```python
from build123d import *

# Parameters (mm, degrees)
SKETCH4_W          = 3.175
SKETCH4_H          = 3.175
CUT_EXTRUDE2_DEPTH = 40.272581084
SKETCH5_R          = 1.5875
CUT_EXTRUDE3_DEPTH = 40.272581084
FILLET1_R          = 1.27


with BuildPart() as part:
    # Sketch3 → Revolve2 (revolve)
    with BuildSketch(Plane(origin=(0, 0, 0), x_dir=(0, 0, -1), z_dir=(1, 0, 0)), mode=Mode.PRIVATE) as revolve2_sk:
        Polygon((0, 6.35), (28.575, 6.35), (28.575, 19.05), (26.9875, 19.05), (22.225, 11.1125), (19.05, 11.1125), (14.2875, 19.05), (12.7, 19.05), (12.7, 12.7), (0, 12.7), align=None)
    revolve(revolve2_sk.sketch.rotate(Axis((0, 0, 0), (0, 0, -1)), 90), axis=Axis((0, 0, 0), (0, 0, -1)))

    # Sketch4 → Cut-Extrude2 (cut, through all)
    with BuildSketch(Plane.XY):
        with Locations((0, 6.35)):
            Rectangle(SKETCH4_W, SKETCH4_H)
    extrude(amount=-CUT_EXTRUDE2_DEPTH, mode=Mode.SUBTRACT)

    # Sketch5 → Cut-Extrude3 (cut, through all)
    with BuildSketch(Plane(origin=(0, 0, 0), x_dir=(1, 0, 0), z_dir=(0, 1, 0))):
        with Locations(Location((0, 6.35, 0), (0, 0, 90))):
            Circle(SKETCH5_R)
    extrude(amount=CUT_EXTRUDE3_DEPTH, mode=Mode.SUBTRACT)

    # Fillet1
    fillet1_edges = [part.edges().sort_by_distance(p)[0] for p in [
        (-12.7, 0, -12.7),
        (-12.7, 0, 0),
    ]]
    fillet(fillet1_edges, radius=FILLET1_R)


solid = part.part
```
Geometry: final body of the model. Coordinates: model frame, mm. A direction names the side the tool comes from. Coordinates: 2 decimals unless noted, no trailing zeros. Order: outer loops, then holes, each group sorted by start corner. A loop starts at its lowest first (then second) coordinate and runs counter-clockwise, first axis right, second up. Notation, with made-up numbers: (6, 12) - (53, 12) arc R12 cw to (53, 31) - close; hole circle Ø11 at (73.5, 11.5). An arc over 180 degrees is marked (long way). Return JSON: item names as keys, results as strings. Group by question number.
1. Pull-direction query (Y, two-part tool) for faces 6 (the face through (0, 7.938, -2)), 7 (the face through (1.588, 7, -14)), 8 (the face through (-8.2, -7.5, -20.6)), 9 (the face through (-6, -13, -12.7)); classes: pulls with the +Y half, pulls with the -Y half, needs draft (parallel to the pull), parting line crosses it, or undercut.
2. Set-up query: faces 1 (the face through (-9.124, 6.996, -22.456)), 2 (the face through (-10.1, 7.7, -6.3)), 3 (the face through (0.966, 10.287, -5.09)), 4 (the face through (-1.588, 7, -14)), 5 (the face through (5, -5, -28.575)). Return all of +Z, -Z, +X, -X, +Y, -Y with unobstructed straight access to the full face (end or side cutting, diameter ignored); none if empty.
3. Pin query (flat end, axial travel): pin 1 (1.5 mm diameter, centred on x = -6.5, z = -14, fed in from -Y); pin 2 (1 mm diameter, centred on x = 0.5, z = -3, fed in from -Y); pin 3 (10 mm diameter, centred on y = -11.5, z = -6.5, fed in from -X). Return the tip coordinate at first contact, or that it passes through.
4. Material intervals for line 1 along Y through (x, z) = (0, -17.5); line 2 along X through (y, z) = (10.65, -6.35); line 3 along X through (y, z) = (11.6, -6.35), sorted ascending. Write a range as [from, to].
5. Cut plane D-D (z = -13.25). Output: boundary loops of the cut face in (x, y), plus the area to 3 significant figures.
6. Cut plane C-C (z = -9). Output: boundary loops of the cut face in (x, y).
7. Cut plane B-B (x = 0). Count the separate pieces of the cut face and the enclosed holes in it, plus the area to 3 significant figures.
Resolved:
{
 "1": {"face 6": "undercut", "face 7": "undercut", "face 8": "parting line crosses it", "face 9": "needs draft"},
 "2": {"face 1": "none", "face 2": "+Z", "face 3": "+Y", "face 4": "+Z, -Z", "face 5": "-Z, +X, -X, +Y, -Y"},
 "3": {"pin 1": "stops at y = -18.16", "pin 2": "stops at y = -12.7", "pin 3": "stops at x = -10.91"},
 "4": {"line 1": "y = [-13.7, -6.35], [7.94, 13.7]", "line 2": "x = [-6.92, -1.59], [1.59, 6.92]", "line 3": "x = [-5.17, -1.59], [1.59, 5.17]"},
 "5": {"outline": "circle Ø38.1 at (0, 0); hole (-1.59, 6.15) arc R6.35 ccw (long way) to (1.59, 6.15) - (1.59, 7.94) - (-1.59, 7.94) - close", "area": "1,010 mm²"},
 "6": {"outline": "circle Ø25.4 at (0, 0); hole (-1.59, 6.15) arc R6.35 ccw (long way) to (1.59, 6.15) - (1.59, 7.94) - (-1.59, 7.94) - close"},
 "7": {"separate pieces": "3", "enclosed holes": "0", "area": "378 mm²"}
}
